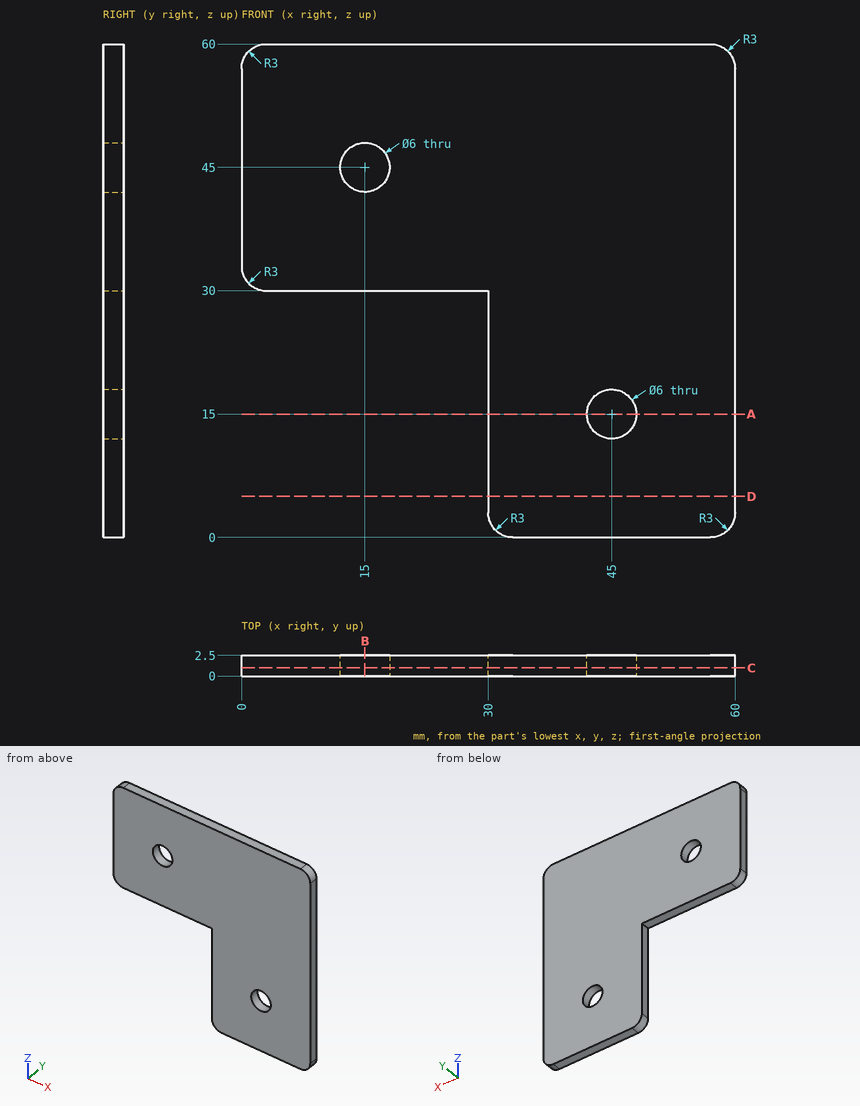
Study the drawing (mm; zero at the part's minimum x, y, z) and answer. Coordinates: 2 decimals unless noted, no trailing zeros. Order: outer loops, then holes, each group sorted by start corner. A loop starts at its lowest first (then second) coordinate and runs counter-clockwise, first axis right, second up. Notation, with made-up numbers: M -14,51 L 21,51 A27 ccw 21,72 Z; hole C 26.5,13 d1. An arc over 180 degrees is marked long. Answer as a JSON object with one key per item and string values. Group by question number.
1. Section A-A on z = 15 is taken. Write down the section's boundary in (x, y), then the cut area to 3 significant figures.
2. Section B-B on x = 15 is taken. Write down the section's boundary in (y, z).
3. Section C-C on y = 1 is taken. Write down the section's boundary in (x, z), then the cut area to 3 significant figures.
4. Flat-ended cylindrical pins translate along their axes: P1, Ø5, axis at x = 15, z = 45, coming from the -Y side; P2, Ø1.5, axis at y = 2, z = 26, coming from the -X side; P3, Ø1.2, axis at x = 13, y = 1, coming from the -Z side; P4, Ø7, axis at x = 45, z = 15, coming from the +Y side. Find the tip coordinate at first contact, or state that the pin passes through.
5. Straight lines are drawn through the part: line 1 (X direction, y = 0.9, z = 45); line 2 (X direction, y = 0.65, z = 15). For each, find the intervals that lie inside material, in ascending order.
6. Section D-D on z = 5 is taken. Write down the section's boundary in (x, y).
Values follow:
{
 "1": {"outline": "M 30,0 L 42,0 L 42,2.5 L 30,2.5 Z; M 48,0 L 60,0 L 60,2.5 L 48,2.5 Z", "area": "60.0 mm2"},
 "2": {"outline": "M 0,30 L 2.5,30 L 2.5,42 L 0,42 Z; M 0,48 L 2.5,48 L 2.5,60 L 0,60 Z"},
 "3": {"outline": "M 0,33 A3 ccw 3,30 L 30,30 L 30,3 A3 ccw 33,0 L 57,0 A3 ccw 60,3 L 60,57 A3 ccw 57,60 L 3,60 A3 ccw 0,57 Z; hole C 15,45 d6; hole C 45,15 d6", "area": "2,630 mm2"},
 "4": {"P1": "through", "P2": "x = 30", "P3": "z = 30", "P4": "y = 2.5"},
 "5": {"line 1": "0 to 12, 18 to 60", "line 2": "30 to 42, 48 to 60"},
 "6": {"outline": "M 30,0 L 60,0 L 60,2.5 L 30,2.5 Z"}
}
